Can you work these out from the model? Positions are in its coordinate system, mm. A direction names the side the tool comes from. Coordinates: 2 decimals unless noted, no trailing zeros. Order: outer loops, then holes, each group sorted by start corner. A loop starts at its lowest first (then second) coordinate and runs counter-clockwise, first axis right, second up. Notation, with made-up numbers: (-10, 34.5) -> (10, 34.5) arc R13 cw to (10, 49.5) -> close; hole circle Ø3 at (31, 41.25). An arc over 180 degrees is marked (long way). Answer in a Markdown table with one row per item.
```python
from build123d import *

# Parameters (mm, degrees)
EXTRUDE_3_DEPTH     = 16
SKETCH_8_R          = 5
CUT_EXTRUDE_3_DEPTH = 190.307289875
SKETCH_9_R          = 6.5
CUT_EXTRUDE_4_DEPTH = 190.307289875
FILLET_1_R          = 10
FILLET_2_R          = 20
FILLET_3_R          = 2
FILLET_4_R          = 10


with BuildPart() as part:
    # 草图1 → 凸台-拉伸3 (new body)
    with BuildSketch(Plane.XY):
        Polygon((52.5, 0), (90, 19), (107.5, 19), (107.5, 39), (90, 39), (52.5, 85), (25, 85), (25, 155), (-25, 155), (-25, 85), (-52.5, 85), (-90, 39), (-107.5, 39), (-107.5, 19), (-90, 19), (-52.5, 0), align=None)
    extrude(amount=EXTRUDE_3_DEPTH)

    # 草图8 → 切除-拉伸3 (cut, through all)
    with BuildSketch(Plane.XY.offset(16)):
        with Locations((-95, 39)):
            Circle(SKETCH_8_R)
        with Locations((-95, 19)):
            Circle(SKETCH_8_R)
        with Locations((95, 39)):
            Circle(SKETCH_8_R)
        with Locations((95, 19)):
            Circle(SKETCH_8_R)
    extrude(amount=-CUT_EXTRUDE_3_DEPTH, mode=Mode.SUBTRACT)

    # 草图9 → 切除-拉伸4 (cut, through all)
    with BuildSketch(Plane.XY.offset(16)):
        with Locations((-50, 40)):
            Circle(SKETCH_9_R)
        with Locations((50, 40)):
            Circle(SKETCH_9_R)
    extrude(amount=-CUT_EXTRUDE_4_DEPTH, mode=Mode.SUBTRACT)

    # 圆角1
    fillet_1_edges = [part.edges().sort_by_distance(p)[0] for p in [
        (-25, 85, 8),
        (25, 85, 8),
    ]]
    fillet(fillet_1_edges, radius=FILLET_1_R)

    # 圆角2
    fillet_2_edges = [part.edges().sort_by_distance(p)[0] for p in [
        (-52.5, 0, 8),
        (52.5, 0, 8),
    ]]
    fillet(fillet_2_edges, radius=FILLET_2_R)

    # 圆角3
    fillet_3_edges = [part.edges().sort_by_distance(p)[0] for p in [
        (-90, 19, 8),
        (-107.5, 19, 8),
        (-107.5, 39, 8),
        (-90, 39, 8),
        (90, 39, 8),
        (107.5, 39, 8),
        (107.5, 19, 8),
        (90, 19, 8),
        (-100, 19, 8),
        (100, 39, 8),
        (100, 19, 8),
        (-100, 39, 8),
    ]]
    fillet(fillet_3_edges, radius=FILLET_3_R)

    # 圆角4
    fillet_4_edges = [part.edges().sort_by_distance(p)[0] for p in [
        (-52.5, 85, 8),
        (52.5, 85, 8),
    ]]
    fillet(fillet_4_edges, radius=FILLET_4_R)


solid = part.part
```
(1) Suppose I cut it at B-B (y = 106). Please give me the cut outline in (x, z), and give its area (3 significant figures).
Response values:
| item | result |
|---|---|
| outline | (-25, 0) -> (25, 0) -> (25, 16) -> (-25, 16) -> close |
| area | 800 mm2 |
(2) Will these pins go through, and if not, where does the flat tip stop? pin 1 Ø4 at (x, z) = (-31.5, 12.5) entering from -Y; pin 2 Ø4 at (x, z) = (104.5, 11.5) entering from -Y; pin 3 Ø1.9 at (x, z) = (104, 7) entering from +Y; pin 4 Ø5 at (x, z) = (84.5, 14) entering from -Y.
Response values:
| item | result |
|---|---|
| pin 1 | y = 0 |
| pin 2 | y = 19 |
| pin 3 | y = 39 |
| pin 4 | y = 14.95 |
(3) On a 3-axis mill with a long thin cutter (end or side, diameter ignored), from which of +Z, -Z, +X, -X, +Y, -Y can I reach the whole of each face in a straight line? I mean faces 1 (the flat face through (-41, 85, 8)), 2 (the flat face through (41, 85, 8)), 3 (the cylindrical face through (-52.43, 0.56, 8.11)). Say none if no direction works.
Response values:
| item | result |
|---|---|
| face 1 | +Z, -Z, -X, +Y |
| face 2 | +Z, -Z, +X, +Y |
| face 3 | +Z, -Z, -X, -Y |
(4) Suppose I cut it at D-D (x = -85.5). Please give me the cut outline in (y, z).
Response values:
| item | result |
|---|---|
| outline | (16.72, 0) -> (44.52, 0) -> (44.52, 16) -> (16.72, 16) -> close |
(5) Suppose I cut it at C-C (z = 7). Count the separate pieces of the cut face and the enclosed holes in it, and give its area (3 significant figures).
Response values:
| item | result |
|---|---|
| separate pieces | 1 |
| enclosed holes | 2 |
| area | 16,700 mm2 |
(6) I need wall thicknesses on line 1 (Y direction, x = 50, z = 9); line 2 (X direction, y = 124, z = 8.25); line 3 (Y direction, x = -82.5, z = 12.75). Which ranges of each line are inside material? Lowest first, please. Write a range as [from, to].
Response values:
| item | result |
|---|---|
| line 1 | [0.13, 33.5], [46.5, 84.74] |
| line 2 | [-25, 25] |
| line 3 | [15.2, 48.2] |
(7) Suppose I cut it at A-A (x = -50). Please give me the cut outline in (y, z).
Response values:
| item | result |
|---|---|
| outline | (0.13, 0) -> (33.5, 0) -> (33.5, 16) -> (0.13, 16) -> close; (46.5, 0) -> (84.74, 0) -> (84.74, 16) -> (46.5, 16) -> close |
(8) We'd pull the mould along X, two halves only. Please class faces 4 (the cylindrical face through (95, 24, 8)), 5 (the flat face through (72.8, 60.1, 7.9)), 6 (the cylindrical face through (-95, 24, 8)), 7 (the cylindrical face through (-52.097, 84.006, 8.112)): +X half, -X half, draft (parallel to the pull), parting line (faces both ways), or undercut.
Response values:
| item | result |
|---|---|
| face 4 | undercut |
| face 5 | +X half |
| face 6 | undercut |
| face 7 | -X half |
